```python
from build123d import *

# Parameters (mm, degrees)
SKETCH1_R           = 76.2
BOSS_EXTRUDE1_DEPTH = 6.35
SKETCH2_R           = 1.25
SKETCH2_R_2         = 1.855
CUT_EXTRUDE1_DEPTH  = 108.95
SKETCH3_R           = 1.855
CUT_EXTRUDE2_DEPTH  = 108.95
SKETCH5_R           = 1.25
SKETCH5_R_2         = 1.5
CUT_EXTRUDE3_DEPTH  = 10


with BuildPart() as part:
    # Sketch1 → Boss-Extrude1 (new body)
    with BuildSketch(Plane.XY):
        Circle(SKETCH1_R)
    extrude(amount=BOSS_EXTRUDE1_DEPTH)

    # Sketch2 → Cut-Extrude1 (cut, through all)
    with BuildSketch(Plane.XY.offset(6.35)):
        with Locations((-43.5, 35)):
            Circle(SKETCH2_R)
        with Locations((43.5, 35)):
            Circle(SKETCH2_R)
        with Locations((-43.5, -35)):
            Circle(SKETCH2_R)
        with Locations((43.5, -35)):
            Circle(SKETCH2_R)
        with Locations((17.5, -45)):
            Circle(SKETCH2_R_2)
        with Locations((-17.5, -45)):
            Circle(SKETCH2_R_2)
        with Locations((9, -61)):
            Circle(SKETCH2_R)
        with Locations((-9, -61)):
            Circle(SKETCH2_R)
        with Locations((-9, -55)):
            Circle(SKETCH2_R)
        with Locations((9, -55)):
            Circle(SKETCH2_R)
    extrude(amount=-CUT_EXTRUDE1_DEPTH, mode=Mode.SUBTRACT)

    # Sketch3 → Cut-Extrude2 (cut, through all)
    with BuildSketch(Plane(origin=(0, 0, 0), x_dir=(-1, 0, 0), z_dir=(0, 0, -1))):
        with Locations((-59.85, 11.05)):
            Circle(SKETCH3_R)
        with Locations((-47.15, 11.05)):
            Circle(SKETCH3_R)
        with Locations((-34.45, 11.05)):
            Circle(SKETCH3_R)
        with Locations((-34.45, -11.05)):
            Circle(SKETCH3_R)
        with Locations((-47.15, -11.05)):
            Circle(SKETCH3_R)
        with Locations((-59.85, -11.05)):
            Circle(SKETCH3_R)
    extrude(amount=-CUT_EXTRUDE2_DEPTH, mode=Mode.SUBTRACT)

    # Sketch5 → Cut-Extrude3 (cut)
    with BuildSketch(Plane(origin=(0, 0, 0), x_dir=(-1, 0, 0), z_dir=(0, 0, -1))):
        with Locations((-9, 61)):
            Circle(SKETCH5_R)
        with Locations((-9, 55)):
            Circle(SKETCH5_R)
        with Locations((9, 61)):
            Circle(SKETCH5_R)
        with Locations((9, 55)):
            Circle(SKETCH5_R)
        with Locations((34.45, 11.05)):
            Circle(SKETCH5_R_2)
        with Locations((47.15, 11.05)):
            Circle(SKETCH5_R_2)
        with Locations((59.85, 11.05)):
            Circle(SKETCH5_R_2)
        with Locations((59.85, -11.05)):
            Circle(SKETCH5_R_2)
        with Locations((47.15, -11.05)):
            Circle(SKETCH5_R_2)
        with Locations((34.45, -11.05)):
            Circle(SKETCH5_R_2)
    extrude(amount=-CUT_EXTRUDE3_DEPTH, mode=Mode.SUBTRACT)


solid = part.part
```
For this review, take the finished solid that the model builds, in its own axes (mm). Round coordinates to 2 decimals unless told otherwise and drop trailing zeros. Loops run counter-clockwise (first coordinate to the right, second up) from the corner with the lowest first, then second, coordinate; pieces in that order, holes last.
(1) Mouldability with a two-part tool opening along Y and no side actions: class faces 1 (the cylindrical face through (17.1, -46.81, 3.22)), 2 (the cylindrical face through (-60.47, -46.367, 3.131)), 3 (the flat face through (-1, 1, 6.35)) as released by +Y, released by -Y, zero draft, split by the parting line, or undercut.
Returned:
face 1: undercut
face 2: split by the parting line
face 3: zero draft
(2) We need section D-D (y = 40). Give the boundary of the cut face in (x, z).
Returned:
outline: (-64.86, 0) - (64.86, 0) - (64.86, 6.35) - (-64.86, 6.35) - close
(3) We need section C-C (x = 54). Give the boundary of the cut face in (y, z).
Returned:
outline: (-53.76, 0) - (53.76, 0) - (53.76, 6.35) - (-53.76, 6.35) - close
(4) We need section B-B (y = -45). Give the boundary of the cut face in (x, z) (3 decimals), plus the area to 3 significant figures.
Returned:
outline: (-61.493, 0) - (-19.355, 0) - (-19.355, 6.35) - (-61.493, 6.35) - close; (-15.645, 0) - (15.645, 0) - (15.645, 6.35) - (-15.645, 6.35) - close; (19.355, 0) - (61.493, 0) - (61.493, 6.35) - (19.355, 6.35) - close
area: 734 mm2
(5) We need section A-A (z = 3.25). State how many separate pieces and enclosed holes the cut face has, plus the area to 3 significant figures.
Returned:
separate pieces: 1
enclosed holes: 26
area: 18,100 mm2
(6) Wall thickness on line 1 along Y through (x, z) = (43.5, 2.75); line 2 along Y through (x, z) = (-35.5, 4.75); line 3 along Y through (x, z) = (9, 3.75): over which ranges is each line inside the solid? List them lowest first.
Returned:
line 1: y = -62.56 to -36.25, -33.75 to 33.75, 36.25 to 62.56
line 2: y = -67.43 to -12.12, -9.98 to 9.98, 12.12 to 67.43
line 3: y = -75.67 to -62.25, -59.75 to -56.25, -53.75 to 53.75, 56.25 to 59.75, 62.25 to 75.67
(7) Clearance check with flat-ended pins moving along their axes: P1, Ø3, axis at y = 35.5, z = 5, coming from the -X side; P2, Ø2, axis at y = 46, z = 3.5, coming from the -X side. State where each tip first meets the part, or that it passes through.
Returned:
P1: stops at x = -68.19
P2: stops at x = -61.49
